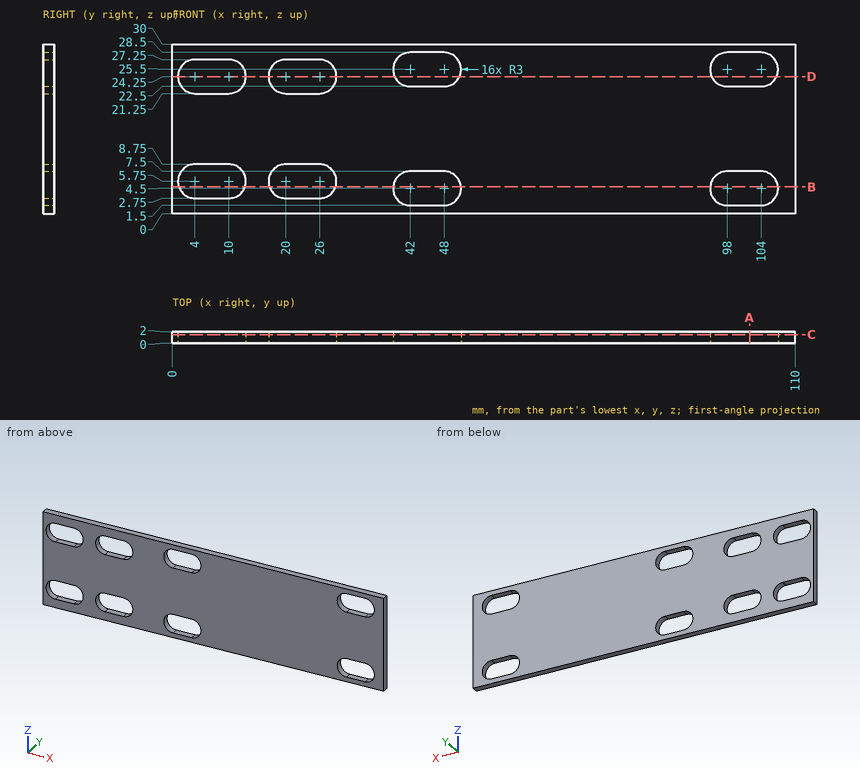
Geometry: see drawing. Coordinates: mm, zero at the bounding-box minimum. Round coordinates to 2 decimals unless told otherwise and drop trailing zeros. Write each loop counter-clockwise with the first axis right and the second up, starting at its lowest first coordinate (ties: lowest second). Pieces come first, ordered by that corner, then holes.
1) Ray query, L1, parallel to Z at x = 102.5, y = 0.4; L2, parallel to Z at x = 5, y = 0.7; L3, parallel to X at y = 1.6, z = 23. Return the intervals inside material, ascending.
2) Cut plane A-A (x = 102). Return the cut outline in (y, z), then the cut area to 3 significant figures.
3) Cut plane C-C (y = 1.5). Count the separate pieces of the cut face and the enclosed holes in it, then the cut area to 3 significant figures.
4) Cut plane B-B (z = 4.75). Return the cut outline in (x, y).
5) Cut plane D-D (z = 24.25). Return the cut outline in (x, y), then the cut area to 3 significant figures.
Geometry says:
1. L1: z = 0 to 1.5, 7.5 to 22.5, 28.5 to 30
1. L2: z = 0 to 2.75, 8.75 to 21.25, 27.25 to 30
1. L3: x = 0 to 1.27, 12.73 to 17.27, 28.73 to 40.34, 49.66 to 96.34, 105.66 to 110
2. outline: (0, 0) - (2, 0) - (2, 1.5) - (0, 1.5) - close; (0, 7.5) - (2, 7.5) - (2, 22.5) - (0, 22.5) - close; (0, 28.5) - (2, 28.5) - (2, 30) - (0, 30) - close
2. area: 36.0 mm2
3. separate pieces: 1
3. enclosed holes: 8
3. area: 2,790 mm2
4. outline: (0, 0) - (1.17, 0) - (1.17, 2) - (0, 2) - close; (12.83, 0) - (17.17, 0) - (17.17, 2) - (12.83, 2) - close; (28.83, 0) - (39.01, 0) - (39.01, 2) - (28.83, 2) - close; (50.99, 0) - (95.01, 0) - (95.01, 2) - (50.99, 2) - close; (106.99, 0) - (110, 0) - (110, 2) - (106.99, 2) - close
5. outline: (0, 0) - (1, 0) - (1, 2) - (0, 2) - close; (13, 0) - (17, 0) - (17, 2) - (13, 2) - close; (29, 0) - (39.27, 0) - (39.27, 2) - (29, 2) - close; (50.73, 0) - (95.27, 0) - (95.27, 2) - (50.73, 2) - close; (106.73, 0) - (110, 0) - (110, 2) - (106.73, 2) - close
5. area: 126 mm2
